Autodesk Inventor part; units mm, degrees
ref_plane "YZ Plane" through (0, 0, 0) normal (1, 0, 0) x (0, 1, 0)
ref_plane "XZ Plane" through (0, 0, 0) normal (0, 1, 0) x (-1, 0, 0)
ref_plane "XY Plane" through (0, 0, 0) normal (0, 0, 1) x (1, 0, 0)
sketch "Sketch1" plane through (0, 0, 0) normal (0, 0, 1) x (1, 0, 0)
  circle A0 centre (-5, 3.0188) radius 1.5
  circle A1 centre (-15, 3.0188) radius 1.5
  line L0 (0, -36.4812) -> (-20, -36.4812)
  line L1 (-20, -36.4812) -> (-20, 10.5188)
  line L2 (-20, 10.5188) -> (0, 10.5188)
  line L3 (0, 10.5188) -> (0, -36.4812)
  dimension "d0" = 3
  dimension "d1" = 3
  dimension "d2" = 10
  dimension "d3" = 20
  dimension "d4" = 7.5
  dimension "d5" = 7.5
  dimension "d6" = 5
  dimension "d7" = 47
extrude "Extrusion1" add sketch "Sketch1" along normal blind 7
sketch "Sketch2" plane through (-20, -36.4812, 0) normal (0, -1, 0) x (1, 0, 0)
  line L0 (0, 0) -> (0, 7)
  line L1 (0, 0) -> (20, 0)
  line L2 (20, 0) -> (20, 30)
  line L3 (20, 30) -> (0, 30)
  line L4 (0, 30) -> (0, 0)
  circle A0 centre (15, 20) radius 2.25
  circle A1 centre (5, 20) radius 2.25
  dimension "d10" = 30
  dimension "d11" = 4.5
  dimension "d12" = 4.5
  dimension "d13" = 10
  dimension "d14" = 5
  dimension "d15" = 10
extrude "Extrusion2" add sketch "Sketch2" against normal blind 7
equation "\"d5\" = d4"
equation "\"d12\" = d11"
properties part number "EndSwitchBracket"
Check sheet for the modelled part. Datum: model origin and axes. Units: mm. A direction names the side the tool comes from. Round coordinates to 2 decimals unless told otherwise and drop trailing zeros. Loops run counter-clockwise (first coordinate to the right, second up) from the corner with the lowest first, then second, coordinate; pieces in that order, holes last. Notation, with made-up numbers: M -27.75,76 L 12.25,76 A26 ccw 12.25,97 Z; hole C 75,62.25 d4. An arc over 180 degrees is marked long. One line per question, with ' | ' between items. Start each with the question number.
Item 1: Set-up check for faces 1 (the face through (-5.488, -33.03, 17.804)), 2 (the face through (-10, -9, 7)): record each of +Z, -Z, +X, -X, +Y, -Y from which the full face is reachable in a straight line by a thin tool's end or side.
Item 2: Scan lines: probe 1 along Y at (x, z) = (-15, 5.75); probe 2 along Z at (x, y) = (-5, -31); probe 3 along Y at (x, z) = (-18.5, 16). Record each from-to range of solid material in increasing order.
Item 3: Release check for a two-part mould opening along X. For faces 3 (the face through (-10, -29.481, 19)), 4 (the face through (0, -18, 6)), 5 (the face through (-16.5, 3, 3.5)) record: released by +X, released by -X, zero draft, split by the parting line, or undercut.
Item 4: Section check A-A (x = -5). Record the boundary of the cut face in (y, z).
Item 5: Section check C-C (y = -32.5). Record the boundary of the cut face in (x, z), and give its area (3 significant figures).
Item 6: Section check B-B (z = 20). Record the boundary of the cut face in (x, y), and give its area (3 significant figures).
Item 7: Section check D-D (x = -14.25). Record the boundary of the cut face in (y, z), and give its area (3 significant figures).
Item 8: Gauge pin test, flat ends, axial feed: pin 1 Ø4 at (x, z) = (-15, 20) entering from -Y; pin 2 Ø5 at (x, z) = (-14, 12) entering from +Y; pin 3 Ø1.5 at (x, y) = (-8, 4.5) entering from +Z. Record the tip position at first contact, or that the pin passes through.
Worked out:
1) face 1: +Y, -Y | face 2: +Z, +X, -X, +Y
2) probe 1: -36.48 to 1.52, 4.52 to 10.52 | probe 2: 0 to 17.75, 22.25 to 30 | probe 3: -36.48 to -29.48
3) face 3: zero draft | face 4: released by +X | face 5: undercut
4) outline: M -36.48,0 L 1.52,0 L 1.52,7 L -29.48,7 L -29.48,17.75 L -36.48,17.75 Z; M -36.48,22.25 L -29.48,22.25 L -29.48,30 L -36.48,30 Z; M 4.52,0 L 10.52,0 L 10.52,7 L 4.52,7 Z
5) outline: M -20,0 L 0,0 L 0,30 L -20,30 Z; hole C -15,20 d4.5; hole C -5,20 d4.5 | area: 568 mm^2
6) outline: M -20,-36.48 L -17.25,-36.48 L -17.25,-29.48 L -20,-29.48 Z; M -12.75,-36.48 L -7.25,-36.48 L -7.25,-29.48 L -12.75,-29.48 Z; M -2.75,-36.48 L 0,-36.48 L 0,-29.48 L -2.75,-29.48 Z | area: 77.0 mm^2
7) outline: M -36.48,0 L 1.72,0 L 1.72,7 L -29.48,7 L -29.48,17.88 L -36.48,17.88 Z; M -36.48,22.12 L -29.48,22.12 L -29.48,30 L -36.48,30 Z; M 4.32,0 L 10.52,0 L 10.52,7 L 4.32,7 Z | area: 442 mm^2
8) pin 1: through | pin 2: y = -29.48 | pin 3: z = 7
